```python
from build123d import *

# Parameters (mm, degrees)
F0_W   = 38.9583557844
F0_H   = 75.9382499057
F0_W_2 = 6.5562282689
F0_H_2 = 11.2140998244
F0_W_3 = 6.6408021376
F0_H_3 = 14.4509151578


with BuildPart() as f1:
    # F0 (on Front) → F1 (revolve)
    with BuildSketch(Plane.XZ):
        with Locations((19.4791778922, 24.6171006164)):
            Rectangle(F0_W, F0_H)
        Polygon((38.9583557844, -13.3520243364), (0, -13.3520243364), (0, -28.2193049788), (6.5562282689, -28.2193049788), align=None)
        Polygon((6.5562282689, -28.2193049788), (0, -28.2193049788), (0, -40.6660549343), (6.5562282689, -40.6660549343), (6.5562282689, -30.708655715), align=None)
        Polygon((9.5987673849, -30.708655715), (6.5562282689, -30.708655715), (6.5562282689, -40.6660549343), (6.5562282689, -71.4942961931), (6.5562282689, -82.7083960176), (9.5987673849, -82.7083960176), align=None)
        with Locations((3.2781141344, -77.1013461053)):
            Rectangle(F0_W_2, F0_H_2)
        Polygon((6.5562282689, -82.7083960176), (0, -82.7083960176), (0, -85.6381952763), (6.6408021376, -85.6381952763), (9.5987673849, -85.6381952763), (9.5987673849, -82.7083960176), align=None)
        with Locations((3.3204010688, -92.8636528552)):
            Rectangle(F0_W_3, F0_H_3)
        Polygon((6.6408021376, -100.0891104341), (0, -100.0891104341), (0, -123.1093853712), (10.5840368196, -123.1093853712), align=None)
    revolve(axis=Axis((0, 0, -39.0329621732), (0, 0, -1)))


with BuildPart() as f1_1:
    # F2: moved
    add(f1.part.moved(Location((0, 254, 0))))


solid = f1_1.part
```
The listing builds one solid part. Answer for the finished solid, in the listing's coordinates (mm). A direction names the side the tool comes from. Coordinates: 2 decimals unless noted, no trailing zeros. Write each loop counter-clockwise with the first axis right and the second up, starting at its lowest first coordinate (ties: lowest second). Pieces come first, ordered by that corner, then holes. Notation, with made-up numbers: (-13, -13.75) -> (0, -13.75) arc R17 cw to (0, 2.25) -> close; hole circle Ø3 at (64, 24). An arc over 180 degrees is marked (long way). Write each question's results on one line, items separated by ' | '. Start each with the question number.
1) Straight lines are drawn through the part: probe 1 along X at (y, z) = (254, -58); probe 2 along Y at (x, z) = (0, -64.5); probe 3 along X at (y, z) = (288, 16). For each, find the intervals that lie inside material, in ascending order.
2) For a pull along Z with two mould halves and no side action, classify faces 1 (the cylindrical face through (-8.45, 292.03, 25.15)), 2 (the cylindrical face through (-1.42, 260.4, -29.45)), 3 (the flat face through (0, 254, -123.109)), 4 (the conical face through (-1.77, 261.95, -108.88)) as +Z half, -Z half, draft (parallel to the pull), parting line (faces both ways), or undercut.
3) A cutting plane is placed at A-A (y = 254). Determine the outline of the cut face in (x, z), then the cut area to 3 significant figures.
4) A cutting plane is placed at B-B (x = 0). Determine the outline of the cut face in (y, z), then the cut area to 3 significant figures.
5) A cutting plane is placed at C-C (z = -92). Determine the outline of the cut face in (x, y).
6) Flat-ended cylindrical pins translate along their axes: pin 1 Ø6 at (y, z) = (263, -71.5) entering from -X; pin 2 Ø5 at (x, z) = (-0.5, -54.5) entering from -Y; pin 3 Ø5 at (x, z) = (-9.5, -93) entering from +Y; pin 4 Ø3 at (y, z) = (278.5, -13) entering from +X. Find the tip coordinate at first contact, or state that the pin passes through.
7) A cutting plane is placed at D-D (z = 34). Determine the outline of the cut face in (x, y).
8) A tool of negligible diameter and unlimited length cuts with its end or side. For faces 5 (the cylindrical face through (-2.08, 263.37, -57.79)), 6 (the flat face through (1, 253, 62.586)), from which of +Z, -Z, +X, -X, +Y, -Y can it reach the whole face along a straight path? Write none if from no direction.
Values follow:
1) probe 1: -9.6 to -6.56, 6.56 to 9.6 | probe 2: 244.4 to 247.44, 260.56 to 263.6 | probe 3: -19.02 to 19.02
2) face 1: draft | face 2: undercut | face 3: -Z half | face 4: undercut
3) outline: (-38.96, -13.35) -> (-6.56, -28.22) -> (-6.56, -30.71) -> (-9.6, -30.71) -> (-9.6, -85.64) -> (-6.64, -85.64) -> (-6.64, -100.09) -> (-10.58, -123.11) -> (10.58, -123.11) -> (6.64, -100.09) -> (6.64, -85.64) -> (9.6, -85.64) -> (9.6, -30.71) -> (6.56, -30.71) -> (6.56, -28.22) -> (38.96, -13.35) -> (38.96, 62.59) -> (-38.96, 62.59) -> close; hole (-6.56, -71.49) -> (6.56, -71.49) -> (6.56, -40.67) -> (-6.56, -40.67) -> close | area: 7,860 mm²
4) outline: (215.04, -13.35) -> (247.44, -28.22) -> (247.44, -30.71) -> (244.4, -30.71) -> (244.4, -85.64) -> (247.36, -85.64) -> (247.36, -100.09) -> (243.42, -123.11) -> (264.58, -123.11) -> (260.64, -100.09) -> (260.64, -85.64) -> (263.6, -85.64) -> (263.6, -30.71) -> (260.56, -30.71) -> (260.56, -28.22) -> (292.96, -13.35) -> (292.96, 62.59) -> (215.04, 62.59) -> close; hole (247.44, -71.49) -> (260.56, -71.49) -> (260.56, -40.67) -> (247.44, -40.67) -> close | area: 7,860 mm²
5) outline: circle Ø13.28 at (0, 254)
6) pin 1: x = -7.49 | pin 2: y = 244.4 | pin 3: through | pin 4: x = 31.44
7) outline: circle Ø77.92 at (0, 254)
8) face 5: none | face 6: +Z, +X, -X, +Y, -Y
